Work out the finished part from the listing and answer in its coordinate system (mm). Face numbers are marked on the shaded views. Round coordinates to 2 decimals unless told otherwise and drop trailing zeros. Write each loop counter-clockwise with the first axis right and the second up, starting at its lowest first coordinate (ties: lowest second). Pieces come first, ordered by that corner, then holes. Notation, with made-up numbers: (35.5, 49) -> (87.5, 49) arc R8 ccw to (87.5, 58) -> close; hole circle Ø10 at (51, 69.25). An arc over 180 degrees is marked (long way). One line per item, written item: value.
```python
from build123d import *

# Parameters (mm, degrees)
SKETCH_1_W          = 50
SKETCH_1_H          = 50
SKETCH_1_R          = 2.5
EXTRUDE_1_DEPTH     = 14
SKETCH_2_R          = 11.5
CUT_EXTRUDE_1_DEPTH = 58.628118137


with BuildPart() as part:
    # 草图1 → 凸台-拉伸1 (new body)
    with BuildSketch(Plane(origin=(0, 0, 0), x_dir=(1, 0, 0), z_dir=(0, 1, 0))):
        Rectangle(SKETCH_1_W, SKETCH_1_H)
        with Locations(Location((-17.5, 17.5, 0), (0, 0, 270))):
            Circle(SKETCH_1_R, mode=Mode.SUBTRACT)
        with Locations(Location((-17.5, -17.5, 0), (0, 0, 270))):
            Circle(SKETCH_1_R, mode=Mode.SUBTRACT)
        with Locations(Location((17.5, 17.5, 0), (0, 0, 270))):
            Circle(SKETCH_1_R, mode=Mode.SUBTRACT)
        with Locations(Location((17.5, -17.5, 0), (0, 0, 270))):
            Circle(SKETCH_1_R, mode=Mode.SUBTRACT)
    extrude(amount=EXTRUDE_1_DEPTH)

    # 草图2 → 切除-拉伸1 (cut, through all)
    with BuildSketch(Plane.ZY.offset(25)):
        Circle(SKETCH_2_R)
    extrude(amount=-CUT_EXTRUDE_1_DEPTH, mode=Mode.SUBTRACT)


solid = part.part
```
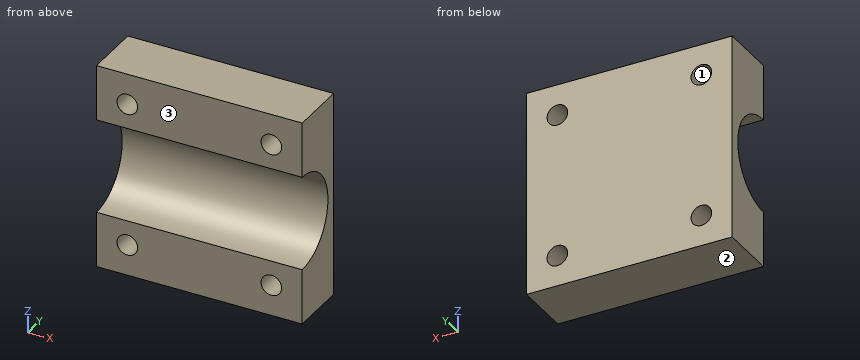
(1) Find section B-B on y = 7. Give the vertices of the cut face in (x, z).
Reported:
outline: (-25, -25) -> (25, -25) -> (25, -9.12) -> (-25, -9.12) -> close; (-25, 9.12) -> (25, 9.12) -> (25, 25) -> (-25, 25) -> close; hole circle Ø5 at (-17.5, -17.5); hole circle Ø5 at (-17.5, 17.5); hole circle Ø5 at (17.5, -17.5); hole circle Ø5 at (17.5, 17.5)
(2) Flat-ended cylindrical pins translate along their axes: pin 1 Ø10 at (x, z) = (-4.5, 1) entering from -Y; pin 2 Ø12 at (x, z) = (10.5, -3.5) entering from -Y. Find the tip coordinate at first contact, or state that the pin passes through.
Reported:
pin 1: stops at y = 9.81
pin 2: stops at y = 6.48
(3) Find section A-A on x = -16. Give the vertices of the cut face in (y, z), plus the area to 3 significant figures.
Reported:
outline: (0, -25) -> (14, -25) -> (14, -19.5) -> (0, -19.5) -> close; (0, -15.5) -> (14, -15.5) -> (14, 15.5) -> (0, 15.5) -> (0, 11.5) arc R11.5 cw to (0, -11.5) -> close; (0, 19.5) -> (14, 19.5) -> (14, 25) -> (0, 25) -> close
area: 380 mm2
(4) Find section D-D on x = 17.5. Give the vertices of the cut face in (y, z).
Reported:
outline: (0, -25) -> (14, -25) -> (14, -20) -> (0, -20) -> close; (0, -15) -> (14, -15) -> (14, 15) -> (0, 15) -> (0, 11.5) arc R11.5 cw to (0, -11.5) -> close; (0, 20) -> (14, 20) -> (14, 25) -> (0, 25) -> close
(5) Consider probe 1 along X at (y, z) = (7, 17.5); probe 2 along X at (y, z) = (9, 18); probe 3 along Z at (x, y) = (-16.5, 6.25). Determine where each line is inside the solid, lowest interval first.
Reported:
probe 1: x = -25 to -20, -15 to 15, 20 to 25
probe 2: x = -25 to -19.95, -15.05 to 15.05, 19.95 to 25
probe 3: z = -25 to -19.79, -15.21 to -9.65, 9.65 to 15.21, 19.79 to 25
(6) Find section C-C on z = -17.5. Give the vertices of the cut face in (x, y), plus the area to 3 significant figures.
Reported:
outline: (-25, 0) -> (-20, 0) -> (-20, 14) -> (-25, 14) -> close; (-15, 0) -> (15, 0) -> (15, 14) -> (-15, 14) -> close; (20, 0) -> (25, 0) -> (25, 14) -> (20, 14) -> close
area: 560 mm2
(7) For a pull along Z with two mould halves and no side action, classify the marked faces 1, 2 and 3 as pulls with the +Z half, pulls with the -Z half, needs draft (parallel to the pull), parting line crosses it, or undercut.
Reported:
face 1: undercut
face 2: pulls with the -Z half
face 3: needs draft
